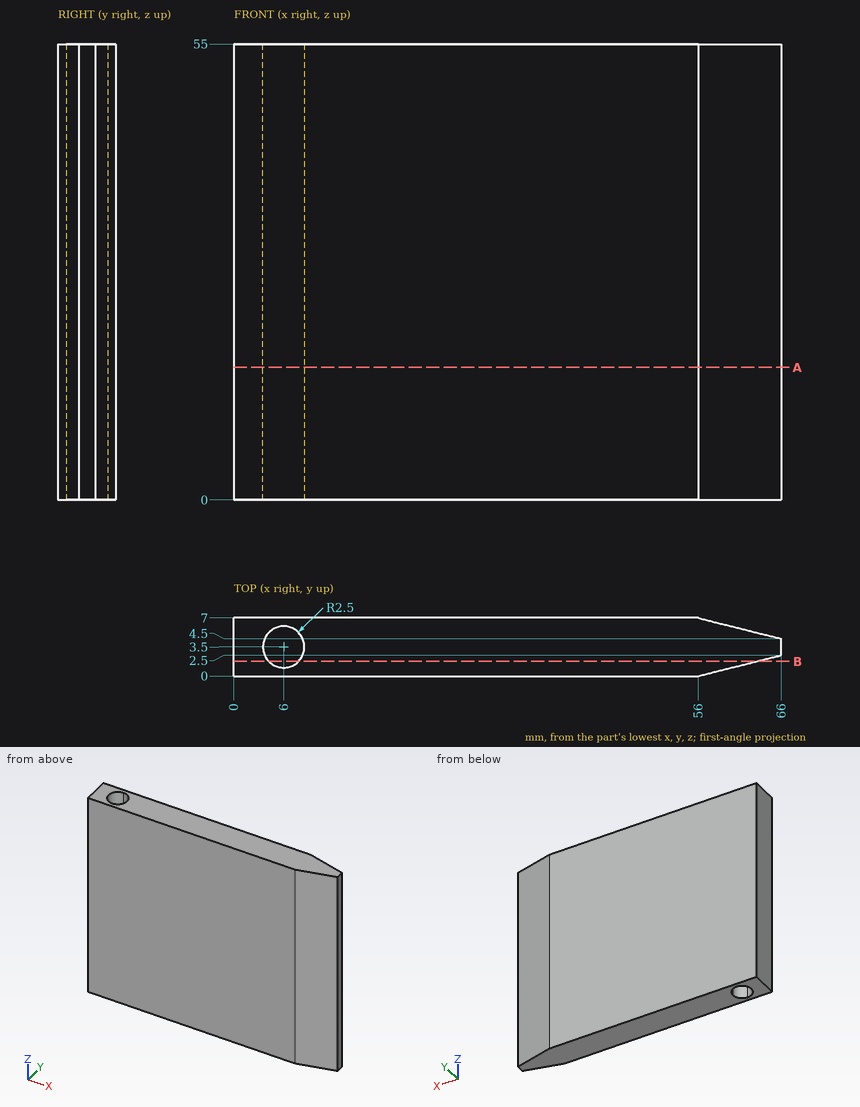
Geometry check sheet. Reference: drawing and pictorial views, mm from the part's lowest x, y, z. Give positions to 0.01 mm unless a question says otherwise; leave off trailing zeros. Order: outer loops, then holes, each group sorted by start corner. A loop starts at its lowest first (then second) coordinate and runs counter-clockwise, first axis right, second up. Notation, with made-up numbers: M 85.25,72 L 113.25,72 A37 ccw 113.25,111 Z; hole C 23,18.25 d5. An arc over 180 degrees is marked long. Use one line per item in the form item = value. Start each with the question number.
Q1. Section check A-A (z = 16). Enter the section's corners in (x, y).
Q2. Go/stop test with a flat-tipped pin: pin 1 Ø3 at (x, y) = (19.5, 3) entering from -Z. Record where the tip stops, or that it passes through.
Q3. Scan lines: line 1 along X through (y, z) = (3.5, 33); line 2 along Y through (x, z) = (61.5, 45) (3 decimals); line 3 along Y through (x, z) = (63.5, 35.5) (3 decimals). Record each from-to range of solid material in increasing order. Write a range as [from, to].
Q4. Section check B-B (y = 1.75). Enter the section's corners in (x, z), then the cut area to 3 significant figures.
Evaluation:
q1.outline = M 0,0 L 56,0 L 66,2.5 L 66,4.5 L 56,7 L 0,7 Z; hole C 6,3.5 d5
q2.pin_1 = 0
q3.line_1 = [0, 3.5], [8.5, 66]
q3.line_2 = [1.375, 5.625]
q3.line_3 = [1.875, 5.125]
q4.outline = M 0,0 L 4.21,0 L 4.21,55 L 0,55 Z; M 7.79,0 L 63,0 L 63,55 L 7.79,55 Z
q4.area = 3,270 mm2
